from build123d import *

# Parameters (mm, degrees)
DODANIE_WYCI_GNI_CIE1_DEPTH = 720
WYTNIJ_WYCI_GNI_CIE1_DEPTH  = 729.834686332


with BuildPart() as part:
    # Szkic1 → Dodanie-wyciągnięcie1 (new body)
    with BuildSketch(Plane.XY):
        with BuildLine():
            Line((8, 0), (72, 0))
            ThreePointArc((72, 0), (77.656854249, 2.343145751), (80, 8))
            Line((80, 8), (80, 72))
            ThreePointArc((80, 72), (77.656854249, 77.656854249), (72, 80))
            Line((72, 80), (8, 80))
            ThreePointArc((8, 80), (2.343145751, 77.656854249), (0, 72))
            Line((0, 72), (0, 8))
            ThreePointArc((0, 8), (2.343145751, 2.343145751), (8, 0))
        make_face()
        with BuildLine():
            Line((5, 8), (5, 72))
            ThreePointArc((5, 72), (5.878679656, 74.121320344), (8, 75))
            Line((8, 75), (72, 75))
            ThreePointArc((72, 75), (74.121320344, 74.121320344), (75, 72))
            Line((75, 72), (75, 8))
            ThreePointArc((75, 8), (74.121320344, 5.878679656), (72, 5))
            Line((72, 5), (8, 5))
            ThreePointArc((8, 5), (5.878679656, 5.878679656), (5, 8))
        make_face(mode=Mode.SUBTRACT)
    extrude(amount=-DODANIE_WYCI_GNI_CIE1_DEPTH)

    # Szkic2 → Wytnij-wyciągnięcie1 (cut, through all)
    with BuildSketch(Plane(origin=(0, 80, 0), x_dir=(1, 0, 0), z_dir=(0, 1, 0))):
        Polygon((0, 0), (80, 0), (80, 80), align=None)
        Polygon((80, 640), (0, 720), (80, 720), align=None)
    extrude(amount=-WYTNIJ_WYCI_GNI_CIE1_DEPTH, mode=Mode.SUBTRACT)


solid = part.part
Build history of the part. All positions in model axes, mm. A direction names the side the tool comes from. Coordinates: 2 decimals unless noted, no trailing zeros. Write each loop counter-clockwise with the first axis right and the second up, starting at its lowest first coordinate (ties: lowest second). Pieces come first, ordered by that corner, then holes. Notation, with made-up numbers: (-37, 22.25) -> (-8, 22.25) arc R34 ccw to (-8, 53.25) -> close; hole circle Ø1 at (70, 74.25). An arc over 180 degrees is marked (long way). Use CSV: the item, a comma, the result in double quotes. Start each with the question number.
Q1. Flat gauge pin, fed straight in: pin 1 Ø1.5 at (y, z) = (11, -646) entering from +X. Where does the tip first touch, or does it go through?
Q2. 3-axis set-ups, long thin cutter, end or side, ignore diameter. For faces 1 (the flat face through (40, 5, -355)), 2 (the flat face through (40, 76, -680)): which of +Z, -Z, +X, -X, +Y, -Y reach the whole face in a straight line?
Q3. Cut at A-A, the plane x = 50. List the corners of the cut face in (y, z), then the cut area to 3 significant figures.
Q4. Cut at C-C, the plane z = -543. List the corners of the cut face in (x, y).
Q5. Cut at B-B, the plane y = 45. List the corners of the cut face in (x, z).
Q6. Pull direction Y, two halves, no side cores. Call faces 3 (the flat face through (80, 40, -356)), 4 (the flat face through (75, 40, -356)), 5 (the flat face through (40, 80, -355)): released by +Y, released by -Y, zero draft, split by the parting line, or undercut.
Q7. Drill centre lines: probe 1 along X at (y, z) = (68.5, -149.5); probe 2 along X at (y, z) = (6.5, -469.5). Where is each one in solid material? Low to high.
Checked values:
1,pin 1,"stops at x = 5"
2,face 1,"+Z, -Z"
2,face 2,"-Z, +X, +Y, -Y"
3,outline,"(0, -670) -> (5, -670) -> (5, -50) -> (0, -50) -> close; (75, -670) -> (80, -670) -> (80, -50) -> (75, -50) -> close"
3,area,"6,200 mm²"
4,outline,"(0, 8) arc R8 ccw to (8, 0) -> (72, 0) arc R8 ccw to (80, 8) -> (80, 72) arc R8 ccw to (72, 80) -> (8, 80) arc R8 ccw to (0, 72) -> close; hole (5, 8) arc R3 ccw to (8, 5) -> (72, 5) arc R3 ccw to (75, 8) -> (75, 72) arc R3 ccw to (72, 75) -> (8, 75) arc R3 ccw to (5, 72) -> close"
5,outline,"(0, -720) -> (5, -715) -> (5, -5) -> (0, 0) -> close; (75, -645) -> (80, -640) -> (80, -80) -> (75, -75) -> close"
6,face 3,"zero draft"
6,face 4,"undercut"
6,face 5,"released by +Y"
7,probe 1,"x = 0 to 5, 75 to 80"
7,probe 2,"x = 0.14 to 5.4, 74.6 to 79.86"
